```python
from build123d import *

# Parameters (mm, degrees)
F0_W     = 110
F0_H     = 56
F1_DEPTH = 3.6
F2_T     = -0.5


with BuildPart() as f1:
    # F0 (on Right) → F1 (new body, symmetric)
    with BuildSketch(Plane.YZ):
        Rectangle(F0_W, F0_H)
    extrude(amount=F1_DEPTH, both=True)

    # F2
    f2_openings = [f1.faces().sort_by_distance(p)[0] for p in [
        (0, -55, 0),
    ]]
    offset(amount=F2_T, openings=f2_openings)


solid = f1.part
```
Can you work these out from the model? Positions are in its coordinate system, mm. A direction names the side the tool comes from. Give positions to 0.01 mm unless a question says otherwise; leave off trailing zeros. Order: outer loops, then holes, each group sorted by start corner. A loop starts at its lowest first (then second) coordinate and runs counter-clockwise, first axis right, second up. Notation, with made-up numbers: M 44.5,61.25 L 57.5,61.25 A21 cw 57.5,91.25 Z; hole C 44,22 d7. An arc over 180 degrees is marked long. Write item = value, one per line. Start each with the question number.
Q1. For faces 1 (the flat face through (-3.4, -55, -0.1)), 2 (the flat face through (0, 54.5, 0)), which set-ups out of +Z, -Z, +X, -X, +Y, -Y let a thin tool reach every point of the face, with its end or its side?
Q2. Suppose I cut it at B-B (z = 21). Write out the boundary of the cut face in (x, y), plus the area to 3 significant figures.
Q3. I need wall thicknesses on probe 1 along Z at (x, y) = (1.5, -13.5); probe 2 along X at (y, z) = (2.5, 6.5); probe 3 along Y at (x, z) = (-1.5, -15). Which ranges of each line are inside material? Lowest first, please. Write a range as [from, to].
Q4. We'd pull the mould along X, two halves only. Please class faces 3 (the flat face through (-3.6, -1, 0)), 4 (the flat face through (0, -1, 27.5)), 5 (the flat face through (3.6, -1, 0)), 6 (the flat face through (0, -1, -28)): pulls with the +X half, pulls with the -X half, needs draft (parallel to the pull), parting line crosses it, or undercut.
Q5. Will this pin go through, and if not, where does the flat tip stop? pin 1 Ø1.5 at (x, z) = (-2, 20.5) entering from -Y.
Q6. Suppose I cut it at A-A (y = 14). Write out the boundary of the cut face in (x, z), plus the area to 3 significant figures.
Q7. Suppose I cut it at C-C (x = 1.25). Write out the boundary of the cut face in (y, z).
Check result:
q1.face_1 = +Z, -Z, +X, -X, -Y
q1.face_2 = -Y
q2.outline = M -3.6,-55 L -3.1,-55 L -3.1,54.5 L 3.1,54.5 L 3.1,-55 L 3.6,-55 L 3.6,55 L -3.6,55 Z
q2.area = 113 mm2
q3.probe_1 = [-28, -27.5], [27.5, 28]
q3.probe_2 = [-3.6, -3.1], [3.1, 3.6]
q3.probe_3 = [54.5, 55]
q4.face_3 = pulls with the -X half
q4.face_4 = undercut
q4.face_5 = pulls with the +X half
q4.face_6 = needs draft
q5.pin_1 = 54.5
q6.outline = M -3.6,-28 L 3.6,-28 L 3.6,28 L -3.6,28 Z; hole M -3.1,-27.5 L 3.1,-27.5 L 3.1,27.5 L -3.1,27.5 Z
q6.area = 62.2 mm2
q7.outline = M -55,-28 L 55,-28 L 55,28 L -55,28 L -55,27.5 L 54.5,27.5 L 54.5,-27.5 L -55,-27.5 Z
